Source: CAD feature listing. Evaluate the final solid. Frame: model axes, mm. Round coordinates to 2 decimals unless told otherwise and drop trailing zeros. Loops run counter-clockwise (first coordinate to the right, second up) from the corner with the lowest first, then second, coordinate; pieces in that order, holes last. Notation, with made-up numbers: (44, 2) -> (103, 2) arc R22 ccw to (103, 37) -> close; hole circle Ø11 at (77, 48.25). An arc over 180 degrees is marked (long way). Write item = value, one per line.
from build123d import *

# Parameters (mm, degrees)
SKETCH1_W                 = 80
SKETCH1_H                 = 80
SKETCH1_R                 = 16
BOSS_EXTRUDE1_DEPTH       = 12.7
CUT_EXTRUDE1_REACH        = 59.977
SKETCH2_R                 = 2.655
FILLET1_R                 = 10
CUT_EXTRUDE2_REACH        = 59.977
SKETCH3_R                 = 2.665
CUT_EXTRUDE3_REACH        = 59.977
FILLET2_R                 = 2.54
FILLET2_OF_MIRROR1_R      = 2.54
CIRPATTERN1_DEPTH         = 12.7
M5X0_8_TAPPED_HOLE1_D     = 4.2
M5X0_8_TAPPED_HOLE1_DEPTH = 5
SKETCH7_R                 = 16
SKETCH7_R_2               = 12.5
BOSS_EXTRUDE2_DEPTH       = 2.5


# Read off the part's stored shape, not the designer's step: CirPattern1
with BuildPart() as part:
    # Sketch1 → Boss-Extrude1 (new body)
    with BuildSketch(Plane(origin=(0, 0, 0), x_dir=(1, 0, 0), z_dir=(0, 1, 0))):
        Rectangle(SKETCH1_W, SKETCH1_H)
        with Locations(Location((0, 0, 0), (0, 0, 270))):
            Circle(SKETCH1_R, mode=Mode.SUBTRACT)
    extrude(amount=BOSS_EXTRUDE1_DEPTH)

    # Sketch2 → Cut-Extrude1 (cut, up to next)
    with BuildSketch(Plane(origin=(0, 12.7, 0), x_dir=(1, 0, 0), z_dir=(0, 1, 0)), mode=Mode.PRIVATE) as cut_extrude1_sk1:
        with Locations(Location((24.748737342, 24.748737342, 0), (0, 0, 270))):
            Circle(SKETCH2_R)
    cut_extrude1_tool1 = extrude(cut_extrude1_sk1.sketch, amount=-CUT_EXTRUDE1_REACH, mode=Mode.PRIVATE) & part.part
    # Sketch2 → Cut-Extrude1 (cut, up to next)
    with BuildSketch(Plane(origin=(0, 12.7, 0), x_dir=(1, 0, 0), z_dir=(0, 1, 0)), mode=Mode.PRIVATE) as cut_extrude1_sk2:
        with Locations(Location((-24.748737342, 24.748737342, 0), (0, 0, 270))):
            Circle(SKETCH2_R)
    cut_extrude1_tool2 = extrude(cut_extrude1_sk2.sketch, amount=-CUT_EXTRUDE1_REACH, mode=Mode.PRIVATE) & part.part
    # Sketch2 → Cut-Extrude1 (cut, up to next)
    with BuildSketch(Plane(origin=(0, 12.7, 0), x_dir=(1, 0, 0), z_dir=(0, 1, 0)), mode=Mode.PRIVATE) as cut_extrude1_sk3:
        with Locations(Location((24.748737342, -24.748737342, 0), (0, 0, 270))):
            Circle(SKETCH2_R)
    cut_extrude1_tool3 = extrude(cut_extrude1_sk3.sketch, amount=-CUT_EXTRUDE1_REACH, mode=Mode.PRIVATE) & part.part
    # Sketch2 → Cut-Extrude1 (cut, up to next)
    with BuildSketch(Plane(origin=(0, 12.7, 0), x_dir=(1, 0, 0), z_dir=(0, 1, 0)), mode=Mode.PRIVATE) as cut_extrude1_sk4:
        with Locations(Location((-24.748737342, -24.748737342, 0), (0, 0, 270))):
            Circle(SKETCH2_R)
    cut_extrude1_tool4 = extrude(cut_extrude1_sk4.sketch, amount=-CUT_EXTRUDE1_REACH, mode=Mode.PRIVATE) & part.part
    add(cut_extrude1_tool1.solids().sort_by_distance((24.748737, 12.7, -24.748737))[0], mode=Mode.SUBTRACT)
    add(cut_extrude1_tool2.solids().sort_by_distance((-24.748737, 12.7, -24.748737))[0], mode=Mode.SUBTRACT)
    add(cut_extrude1_tool3.solids().sort_by_distance((24.748737, 12.7, 24.748737))[0], mode=Mode.SUBTRACT)
    add(cut_extrude1_tool4.solids().sort_by_distance((-24.748737, 12.7, 24.748737))[0], mode=Mode.SUBTRACT)

    # Fillet1
    fillet1_edges = [part.edges().sort_by_distance(p)[0] for p in [
        (40, 6.35, 40),
        (-40, 6.35, 40),
        (-40, 6.35, -40),
        (40, 6.35, -40),
    ]]
    fillet(fillet1_edges, radius=FILLET1_R)

    # Sketch3 → Cut-Extrude2 (cut, up to next)
    with BuildSketch(Plane(origin=(0, 12.7, 0), x_dir=(1, 0, 0), z_dir=(0, 1, 0)), mode=Mode.PRIVATE) as cut_extrude2_sk1:
        with Locations(Location((-30, 30, 0), (0, 0, 270))):
            Circle(SKETCH3_R)
    cut_extrude2_tool1 = extrude(cut_extrude2_sk1.sketch, amount=-CUT_EXTRUDE2_REACH, mode=Mode.PRIVATE) & part.part
    # Sketch3 → Cut-Extrude2 (cut, up to next)
    with BuildSketch(Plane(origin=(0, 12.7, 0), x_dir=(1, 0, 0), z_dir=(0, 1, 0)), mode=Mode.PRIVATE) as cut_extrude2_sk2:
        with Locations(Location((30, 30, 0), (0, 0, 270))):
            Circle(SKETCH3_R)
    cut_extrude2_tool2 = extrude(cut_extrude2_sk2.sketch, amount=-CUT_EXTRUDE2_REACH, mode=Mode.PRIVATE) & part.part
    # Sketch3 → Cut-Extrude2 (cut, up to next)
    with BuildSketch(Plane(origin=(0, 12.7, 0), x_dir=(1, 0, 0), z_dir=(0, 1, 0)), mode=Mode.PRIVATE) as cut_extrude2_sk3:
        with Locations(Location((30, -30, 0), (0, 0, 270))):
            Circle(SKETCH3_R)
    cut_extrude2_tool3 = extrude(cut_extrude2_sk3.sketch, amount=-CUT_EXTRUDE2_REACH, mode=Mode.PRIVATE) & part.part
    # Sketch3 → Cut-Extrude2 (cut, up to next)
    with BuildSketch(Plane(origin=(0, 12.7, 0), x_dir=(1, 0, 0), z_dir=(0, 1, 0)), mode=Mode.PRIVATE) as cut_extrude2_sk4:
        with Locations(Location((-30, -30, 0), (0, 0, 270))):
            Circle(SKETCH3_R)
    cut_extrude2_tool4 = extrude(cut_extrude2_sk4.sketch, amount=-CUT_EXTRUDE2_REACH, mode=Mode.PRIVATE) & part.part
    add(cut_extrude2_tool1.solids().sort_by_distance((-30, 12.7, -30))[0], mode=Mode.SUBTRACT)
    add(cut_extrude2_tool2.solids().sort_by_distance((30, 12.7, -30))[0], mode=Mode.SUBTRACT)
    add(cut_extrude2_tool3.solids().sort_by_distance((30, 12.7, 30))[0], mode=Mode.SUBTRACT)
    add(cut_extrude2_tool4.solids().sort_by_distance((-30, 12.7, 30))[0], mode=Mode.SUBTRACT)

    # Sketch4 → Cut-Extrude3 (cut, up to next)
    with BuildSketch(Plane(origin=(0, 12.7, 0), x_dir=(1, 0, 0), z_dir=(0, 1, 0)), mode=Mode.PRIVATE) as cut_extrude3_sk1:
        with BuildLine():
            Line((-5, 35), (-27.928932188, 35))
            Line((-27.928932188, 35), (-12.259782216, 17.049860411))
            ThreePointArc((-12.259782216, 17.049860411), (-8.03635208, 19.401470183), (-3.387096774, 20.725047055))
            Line((-3.387096774, 20.725047055), (-5, 35))
        make_face()
    cut_extrude3_tool1 = extrude(cut_extrude3_sk1.sketch, amount=-CUT_EXTRUDE3_REACH, mode=Mode.PRIVATE) & part.part
    cut_extrude3 = cut_extrude3_tool1.solids().sort_by_distance((-13.138354, 12.7, -27.973836))[0]
    add(cut_extrude3, mode=Mode.SUBTRACT)

    # Fillet2
    fillet2_edges = [part.edges().sort_by_distance(p)[0] for p in [
        (-12.259782216, 6.35, -17.049860411),
        (-27.928932188, 6.35, -35),
        (-5, 6.35, -35),
        (-3.387096774, 6.35, -20.725047055),
    ]]
    fillet(fillet2_edges, radius=FILLET2_R)

    # Mirror1: Cut-Extrude3 across plane
    add(cut_extrude3.mirror(Plane(origin=(0, 0, 0), x_dir=(0, 0, 1), z_dir=(1, 0, 0))), mode=Mode.SUBTRACT)

    # Fillet2 of Mirror1
    fillet2_of_mirror1_edges = [part.edges().sort_by_distance(p)[0] for p in [
        (12.259782216, 6.35, -17.049860411),
        (27.928932188, 6.35, -35),
        (5, 6.35, -35),
        (3.387096774, 6.35, -20.725047055),
    ]]
    fillet(fillet2_of_mirror1_edges, radius=FILLET2_OF_MIRROR1_R)

    # CirPattern1 outline → CirPattern1 (cut)
    with BuildSketch(Plane(origin=(0, 0, 0), x_dir=(1, 0, 0), z_dir=(0, 1, 0))):
        with BuildLine():
            ThreePointArc((18.176050002, 10.518137018), (19.384019181, 8.078353817), (20.26620798, 5.50280057))
            ThreePointArc((20.26620798, 5.50280057), (21.29044889, 4.067126305), (23.002629913, 3.644437079))
            Line((23.002629913, 3.644437079), (32.745175825, 4.745231161))
            ThreePointArc((32.745175825, 4.745231161), (34.35419463, 5.576946113), (35, 7.269171483))
            Line((35, 7.269171483), (35, 22.340093991))
            ThreePointArc((35, 22.340093991), (33.510928831, 24.652484225), (30.789646778, 24.253603885))
            Line((30.789646778, 24.253603885), (18.704133304, 13.703840627))
            ThreePointArc((18.704133304, 13.703840627), (17.868681187, 12.205709601), (18.176050002, 10.518137018))
        make_face()
        with BuildLine():
            ThreePointArc((-18.176050002, -10.518137018), (-19.384019181, -8.078353817), (-20.26620798, -5.50280057))
            ThreePointArc((-20.26620798, -5.50280057), (-21.29044889, -4.067126305), (-23.002629913, -3.644437079))
            Line((-23.002629913, -3.644437079), (-32.745175825, -4.745231161))
            ThreePointArc((-32.745175825, -4.745231161), (-34.35419463, -5.576946113), (-35, -7.269171483))
            Line((-35, -7.269171483), (-35, -22.340093991))
            ThreePointArc((-35, -22.340093991), (-33.510928831, -24.652484225), (-30.789646778, -24.253603885))
            Line((-30.789646778, -24.253603885), (-18.704133304, -13.703840627))
            ThreePointArc((-18.704133304, -13.703840627), (-17.868681187, -12.205709601), (-18.176050002, -10.518137018))
        make_face()
        with BuildLine():
            ThreePointArc((10.518137018, -18.176050002), (8.078353817, -19.384019181), (5.50280057, -20.26620798))
            ThreePointArc((5.50280057, -20.26620798), (4.067126305, -21.29044889), (3.644437079, -23.002629913))
            Line((3.644437079, -23.002629913), (4.745231161, -32.745175825))
            ThreePointArc((4.745231161, -32.745175825), (5.576946113, -34.35419463), (7.269171483, -35))
            Line((7.269171483, -35), (22.340093991, -35))
            ThreePointArc((22.340093991, -35), (24.652484225, -33.510928831), (24.253603885, -30.789646778))
            Line((24.253603885, -30.789646778), (13.703840627, -18.704133304))
            ThreePointArc((13.703840627, -18.704133304), (12.205709601, -17.868681187), (10.518137018, -18.176050002))
        make_face()
        with BuildLine():
            ThreePointArc((20.26620798, -5.50280057), (19.384019181, -8.078353817), (18.176050002, -10.518137018))
            ThreePointArc((18.176050002, -10.518137018), (17.868681187, -12.205709601), (18.704133304, -13.703840627))
            Line((18.704133304, -13.703840627), (30.789646778, -24.253603885))
            ThreePointArc((30.789646778, -24.253603885), (33.510928831, -24.652484225), (35, -22.340093991))
            Line((35, -22.340093991), (35, -7.269171483))
            ThreePointArc((35, -7.269171483), (34.35419463, -5.576946113), (32.745175825, -4.745231161))
            Line((32.745175825, -4.745231161), (23.002629913, -3.644437079))
            ThreePointArc((23.002629913, -3.644437079), (21.29044889, -4.067126305), (20.26620798, -5.50280057))
        make_face()
        with BuildLine():
            ThreePointArc((-5.50280057, -20.26620798), (-8.078353817, -19.384019181), (-10.518137018, -18.176050002))
            ThreePointArc((-10.518137018, -18.176050002), (-12.205709601, -17.868681187), (-13.703840627, -18.704133304))
            Line((-13.703840627, -18.704133304), (-24.253603885, -30.789646778))
            ThreePointArc((-24.253603885, -30.789646778), (-24.652484225, -33.510928831), (-22.340093991, -35))
            Line((-22.340093991, -35), (-7.269171483, -35))
            ThreePointArc((-7.269171483, -35), (-5.576946113, -34.35419463), (-4.745231161, -32.745175825))
            Line((-4.745231161, -32.745175825), (-3.644437079, -23.002629913))
            ThreePointArc((-3.644437079, -23.002629913), (-4.067126305, -21.29044889), (-5.50280057, -20.26620798))
        make_face()
        with BuildLine():
            ThreePointArc((-20.26620798, 5.50280057), (-19.384019181, 8.078353817), (-18.176050002, 10.518137018))
            ThreePointArc((-18.176050002, 10.518137018), (-17.868681187, 12.205709601), (-18.704133304, 13.703840627))
            Line((-18.704133304, 13.703840627), (-30.789646778, 24.253603885))
            ThreePointArc((-30.789646778, 24.253603885), (-33.510928831, 24.652484225), (-35, 22.340093991))
            Line((-35, 22.340093991), (-35, 7.269171483))
            ThreePointArc((-35, 7.269171483), (-34.35419463, 5.576946113), (-32.745175825, 4.745231161))
            Line((-32.745175825, 4.745231161), (-23.002629913, 3.644437079))
            ThreePointArc((-23.002629913, 3.644437079), (-21.29044889, 4.067126305), (-20.26620798, 5.50280057))
        make_face()
    extrude(amount=CIRPATTERN1_DEPTH, mode=Mode.SUBTRACT)

    # M5x0.8 Tapped Hole1
    with Locations(Plane(origin=(-16.7, 6.35, -40), x_dir=(-1, 0, 0), z_dir=(0, 0, -1))):
        with Locations((0, 0), (-33.5, 0)):
            Hole(M5X0_8_TAPPED_HOLE1_D / 2, depth=M5X0_8_TAPPED_HOLE1_DEPTH)

    # Sketch7 → Boss-Extrude2 (add)
    with BuildSketch(Plane.XZ):
        with Locations(Location((0, 0, 0), (0, 0, 270))):
            Circle(SKETCH7_R)
        with Locations(Location((0, 0, 0), (0, 0, 270))):
            Circle(SKETCH7_R_2, mode=Mode.SUBTRACT)
    extrude(amount=-BOSS_EXTRUDE2_DEPTH)


solid = part.part
1. Mould query, pull axis Y, two halves, no side actions, for faces 1 (the face through (-18.8, 6.4, -37.5)), 2 (the face through (-21.27, 6.26, 4.08)). Classes: released by +Y, released by -Y, zero draft, split by the parting line, or undercut.
Evaluation:
face_1 = undercut
face_2 = zero draft
2. Line query: probe 1 along Z at (x, y) = (-21, 10.25); probe 2 along X at (y, z) = (4.75, -30) (3 decimals); probe 3 along X at (y, z) = (10, 7.5). Output: solid intervals per line, ascending. Write a range as from..to.
Evaluation:
probe_1 = -40..-35, -27.06..-15.71, -4.3..4.3, 15.71..27.06, 35..40
probe_2 = -40..-32.665, -27.335..-23.564, -4.435..4.435, 23.564..27.335, 32.665..40
probe_3 = -40..-35, -19.62..-14.13, 14.13..19.62, 35..40
3. Section query A-A (x = 0). Return the cut outline in (y, z).
Evaluation:
outline = (0, -40) -> (12.7, -40) -> (12.7, -16) -> (2.5, -16) -> (2.5, -12.5) -> (0, -12.5) -> close; (0, 12.5) -> (2.5, 12.5) -> (2.5, 16) -> (12.7, 16) -> (12.7, 40) -> (0, 40) -> close
4. Section query B-B (z = 0). Return the cut outline in (x, y), then the cut area to 3 significant figures.
Evaluation:
outline = (-40, 0) -> (-12.5, 0) -> (-12.5, 2.5) -> (-16, 2.5) -> (-16, 12.7) -> (-40, 12.7) -> close; (12.5, 0) -> (40, 0) -> (40, 12.7) -> (16, 12.7) -> (16, 2.5) -> (12.5, 2.5) -> close
area = 627 mm²
5. Section query C-C (y = 11.5). Give the number of separate pieces and of enclosed holes in the cut face, then the cut area to 3 significant figures.
Evaluation:
separate_pieces = 1
enclosed_holes = 17
area = 3,260 mm²
